Design review of the part built by this model. Coordinates are the model's own, in mm. A direction names the side the tool comes from. Coordinates: 2 decimals unless noted, no trailing zeros. Loops run counter-clockwise (first coordinate to the right, second up) from the corner with the lowest first, then second, coordinate; pieces in that order, holes last. Notation, with made-up numbers: M 59,0 L 104,0 A19 ccw 104,5 Z; hole C -11.75,63 d8. An arc over 180 degrees is marked long. One line per item, written item: value.
```python
from build123d import *

# Parameters (mm, degrees)
SKETCH1_R           = 4.7625
EXTRUDE1_DEPTH      = 44.45
SKETCH2_R           = 6.477
EXTRUDE2_DEPTH      = 3.302
CHAMFER1_SIZE       = 0.6604
EXTRUDE3_DEPTH      = 49.622593123
EXTRUDE3_DEPTH_BACK = 49.622593123
SKETCH3_R           = 1.984375
CHAMFER2_SIZE       = 0.47625


with BuildPart() as part:
    # Sketch1 → Extrude1 (new, symmetric)
    with BuildSketch(Plane.XY):
        Circle(SKETCH1_R)
    extrude(amount=EXTRUDE1_DEPTH, both=True)

    # Sketch2 → Extrude2 (add)
    with BuildSketch(Plane.XY.offset(44.45)):
        with Locations(Location((0, 0, 0), (0, 0, 180))):
            Circle(SKETCH2_R)
    extrude(amount=EXTRUDE2_DEPTH)

    # Chamfer1
    chamfer1_edges = [part.edges().sort_by_distance(p)[0] for p in [
        (6.477, 0, 47.752),
    ]]
    chamfer(chamfer1_edges, length=CHAMFER1_SIZE)

    # Sketch3 → Extrude3 (cut, two sides: drawn at the far end of the back side and taken through both)
    with BuildSketch(Plane(origin=(0, 0, 0), x_dir=(0, 0, -1), z_dir=(1, 0, 0)).offset(-EXTRUDE3_DEPTH_BACK)):
        with Locations(Location((40.084375, 0, 0), (0, 0, 180.000000002))):
            Circle(SKETCH3_R)
    extrude(amount=EXTRUDE3_DEPTH + EXTRUDE3_DEPTH_BACK, mode=Mode.SUBTRACT)

    # Chamfer2
    chamfer2_edges = [part.edges().sort_by_distance(p)[0] for p in [
        (-4.7625, 0, -44.45),
    ]]
    chamfer(chamfer2_edges, length=CHAMFER2_SIZE)


solid = part.part
```
(1) Mouldability with a two-part tool opening along Y and no side actions: class faces 1 (the cylindrical face through (1.404, 6.323, 45.752)), 2 (the cylindrical face through (-0.069, -0.596, -38.192)), 3 (the flat face through (0, 0, -44.45)) as released by +Y, released by -Y, zero draft, split by the parting line, or undercut.
Reply:
face 1: split by the parting line
face 2: undercut
face 3: zero draft
(2) Insertion check: pin 1 (5 mm diameter, centred on y = -2, z = 11, fed in from +X); pin 2 (1.5 mm diameter, centred on x = -3, z = -27, fed in from +Y); pin 3 (2 mm diameter, centred on y = 5, z = 21.5, fed in from -X). Each pin has a flat end and moves straight along its axis. Give the tip position at first contact, or say it passes through.
Reply:
pin 1: stops at x = 4.76
pin 2: stops at y = 4.2
pin 3: stops at x = -2.58
(3) Tool access review of faces 4 (the flat face through (0, 0, 47.752)), 5 (the cylindrical face through (4.543, 1.431, 0.857)): name each direction out of +Z, -Z, +X, -X, +Y, -Y from which nothing blocks a thin tool from reaching the whole face with its end or side.
Reply:
face 4: +Z, +X, -X, +Y, -Y
face 5: -Z
(4) We need section A-A on y = 0. State the section outline as (x, z) points, then the cut area to 3 significant figures.
Reply:
outline: M -6.48,44.45 L -4.76,44.45 L -4.76,-38.1 L 4.76,-38.1 L 4.76,44.45 L 6.48,44.45 L 6.48,47.09 L 5.82,47.75 L -5.82,47.75 L -6.48,47.09 Z; M -4.76,-43.97 L -4.29,-44.45 L 4.29,-44.45 L 4.76,-43.97 L 4.76,-42.07 L -4.76,-42.07 Z
area: 851 mm2
(5) We need section C-C on z = 15.5. State the section outline as (x, y) points (1 decimal), then the cut area to 3 significant figures.
Reply:
outline: C 0,0 d9.5
area: 71.3 mm2
(6) To check wall thickness, follow line 1 along Z through (x, y) = (-2.5, 0); line 2 along Z through (x, y) = (-5, 2.25); line 3 along Z through (x, y) = (-1.5, 1.25). State the ranges of each line that lie inside material, in increasing order. Write a range as [from, to].
Reply:
line 1: z = [-44.45, -42.07], [-38.1, 47.75]
line 2: z = [44.45, 47.75]
line 3: z = [-44.45, -41.63], [-38.54, 47.75]
(7) We need section B-B on x = 0. State the section outline as (y, z) points, then the cut area to 3 significant figures.
Reply:
outline: M -6.48,44.45 L -4.76,44.45 L -4.76,-43.97 L -4.29,-44.45 L 4.29,-44.45 L 4.76,-43.97 L 4.76,44.45 L 6.48,44.45 L 6.48,47.09 L 5.82,47.75 L -5.82,47.75 L -6.48,47.09 Z; hole C 0,-40.08 d3.97
area: 877 mm2
